from build123d import *

# Parameters (mm, degrees)
SKETCH1_W           = 42.418
SKETCH1_H           = 42.418
SKETCH1_R           = 3.175
BOSS_EXTRUDE1_DEPTH = 36.449
BOSS_EXTRUDE2_REACH = 68.815
SKETCH2_W           = 3.175
SKETCH2_H           = 42.418
SKETCH4_W           = 29.523081252
SKETCH4_H           = 25.4
CUT_EXTRUDE2_DEPTH  = 70.020848799
FILLET1_R           = 2.54
FILLET2_R           = 6.35


with BuildPart() as part:
    # Sketch1 → Boss-Extrude1 (new body)
    with BuildSketch(Plane.XY):
        with BuildLine():
            Line((4.064, -24.384), (24.384, -24.384))
            Line((24.384, -24.384), (24.384, 24.384))
            Line((24.384, 24.384), (4.064, 24.384))
            ThreePointArc((4.064, 24.384), (0, 32.512), (-4.064, 24.384))
            Line((-4.064, 24.384), (-24.384, 24.384))
            Line((-24.384, 24.384), (-24.384, -24.384))
            Line((-24.384, -24.384), (-4.064, -24.384))
            ThreePointArc((-4.064, -24.384), (0, -32.512), (4.064, -24.384))
        make_face()
        with BuildLine():
            ThreePointArc((-0.889, 24.384), (0, 30.607), (0.889, 24.384))
            Line((0.889, 24.384), (-0.889, 24.384))
        make_face(mode=Mode.SUBTRACT)
        Rectangle(SKETCH1_W, SKETCH1_H, mode=Mode.SUBTRACT)
        with Locations((0, -27.432)):
            Circle(SKETCH1_R, mode=Mode.SUBTRACT)
    extrude(amount=BOSS_EXTRUDE1_DEPTH)

    # Sketch2 → Boss-Extrude2 (add, up to next)
    with BuildSketch(Plane(origin=(-21.209, 0, 0), x_dir=(0, 0, -1), z_dir=(1, 0, 0)), mode=Mode.PRIVATE) as boss_extrude2_sk1:
        with Locations((-1.5875, 0)):
            Rectangle(SKETCH2_W, SKETCH2_H)
    boss_extrude2_tool1 = extrude(boss_extrude2_sk1.sketch, amount=BOSS_EXTRUDE2_REACH, mode=Mode.PRIVATE) - part.part
    add(boss_extrude2_tool1.solids().sort_by_distance((-21.209, 0, 1.5875))[0])

    # Sketch4 → Cut-Extrude2 (cut, through all)
    with BuildSketch(Plane(origin=(24.384, 0, 0), x_dir=(0, 0, -1), z_dir=(1, 0, 0))):
        with Locations((-21.687459374, 0)):
            Rectangle(SKETCH4_W, SKETCH4_H)
    extrude(amount=-CUT_EXTRUDE2_DEPTH, mode=Mode.SUBTRACT)

    # Fillet1
    fillet1_edges = [part.edges().sort_by_distance(p)[0] for p in [
        (-21.209, -21.209, 19.812),
        (21.209, -21.209, 19.812),
        (21.209, 21.209, 19.812),
        (-21.209, 21.209, 19.812),
        (24.384, 24.384, 18.2245),
        (24.384, -24.384, 18.2245),
        (-24.384, -24.384, 18.2245),
        (-24.384, 24.384, 18.2245),
        (22.7965, 12.7, 6.925918748),
        (22.7965, -12.7, 6.925918748),
        (-22.7965, 12.7, 6.925918748),
        (-22.7965, -12.7, 6.925918748),
    ]]
    fillet(fillet1_edges, radius=FILLET1_R)

    # Fillet2
    fillet2_edges = [part.edges().sort_by_distance(p)[0] for p in [
        (4.064, 24.384, 18.2245),
        (4.064, -24.384, 18.2245),
        (-4.064, -24.384, 18.2245),
        (-4.064, 24.384, 18.2245),
    ]]
    fillet(fillet2_edges, radius=FILLET2_R)


solid = part.part
For this review, take the finished solid that the model builds, in its own axes (mm). A direction names the side the tool comes from. Round coordinates to 2 decimals unless told otherwise and drop trailing zeros. Write each loop counter-clockwise with the first axis right and the second up, starting at its lowest first coordinate (ties: lowest second). Pieces come first, ordered by that corner, then holes. Notation, with made-up numbers: (72, 58) -> (119, 58) arc R28 ccw to (119, 89) -> close; hole circle Ø11 at (13.5, 45). An arc over 180 degrees is marked (long way). Use CSV: the item, a comma, the result in double quotes.
(1) Consider section D-D, the plane z = 4.5. Give the boundary of the cut face in (x, y) (3 decimals), plus the area to 3 significant figures.
Computed values:
outline,"(-24.384, -21.844) arc R2.54 ccw to (-21.844, -24.384) -> (-10.943, -24.384) arc R6.35 cw to (-4.863, -28.9) arc R5.08 ccw to (4.863, -28.9) arc R6.35 cw to (10.943, -24.384) -> (21.844, -24.384) arc R2.54 ccw to (24.384, -21.844) -> (24.384, 21.844) arc R2.54 ccw to (21.844, 24.384) -> (10.943, 24.384) arc R6.35 cw to (4.863, 28.9) arc R5.08 ccw to (-4.863, 28.9) arc R6.35 cw to (-10.943, 24.384) -> (-21.844, 24.384) arc R2.54 ccw to (-24.384, 21.844) -> close; hole (-21.209, -18.669) arc R2.54 ccw to (-18.669, -21.209) -> (18.669, -21.209) arc R2.54 ccw to (21.209, -18.669) -> (21.209, 18.669) arc R2.54 ccw to (18.669, 21.209) -> (-18.669, 21.209) arc R2.54 ccw to (-21.209, 18.669) -> close; hole circle Ø6.35 at (0, -27.432); hole (-0.889, 24.384) -> (0.889, 24.384) arc R3.175 ccw (long way) to start"
area,"684 mm²"
(2) Draft analysis for pull direction Y (two halves, no side actions). For faces 4 (the face through (-23.66, -23.62, 18.48)), 5 (the face through (-23, 0, 6.926)), 6 (the face through (0, -22, 36.449)), state which applies: +Y half, -Y half, draft (parallel to the pull), parting line (faces both ways), or undercut.
Computed values:
face 4,"-Y half"
face 5,"undercut"
face 6,"draft"
(3) Consider section C-C, the plane x = -16. Give the boundary of the cut face in (y, z) (3 decimals), plus the area to 3 significant figures.
Computed values:
outline,"(-24.384, 0) -> (24.384, 0) -> (24.384, 36.449) -> (21.209, 36.449) -> (21.209, 3.175) -> (-21.209, 3.175) -> (-21.209, 36.449) -> (-24.384, 36.449) -> close"
area,"366 mm²"
(4) Consider section A-A, the plane x = 0. Give the boundary of the cut face in (y, z) (3 decimals).
Computed values:
outline,"(-32.512, 0) -> (-30.607, 0) -> (-30.607, 36.449) -> (-32.512, 36.449) -> close; (-24.257, 0) -> (24.384, 0) -> (24.384, 36.449) -> (21.209, 36.449) -> (21.209, 3.175) -> (-21.209, 3.175) -> (-21.209, 36.449) -> (-24.257, 36.449) -> close; (30.607, 0) -> (32.512, 0) -> (32.512, 36.449) -> (30.607, 36.449) -> close"
(5) For faces 1 (the face through (0, 21.209, 20)), 2 (the face through (-16, 24.384, 18)), 3 (the face through (23, -12.7, 23)), list the 3-axis set-ups (+Z, -Z, +X, -X, +Y, -Y) from which the entire face can be reached by the end or side of a thin tool; tool diameter is ignored.
Computed values:
face 1,"+Z"
face 2,"+Z, -Z, -X, +Y"
face 3,"+Z, +X, -X"
(6) To check wall thickness, follow L1, parallel to X at y = -13, z = 24; L2, parallel to Z at x = 2, y = 15 (3 decimals). State the ranges of each line that lie inside material, in increasing order. Write a range as [from, to].
Computed values:
L1,"[-24.38, -21.21], [21.21, 24.38]"
L2,"[0, 3.175]"
(7) Consider section B-B, the plane y = 27.5. Give the boundary of the cut face in (x, z), plus the area to 3 significant figures.
Computed values:
outline,"(-5.48, 0) -> (-3.17, 0) -> (-3.17, 36.45) -> (-5.48, 36.45) -> close; (3.17, 0) -> (5.48, 0) -> (5.48, 36.45) -> (3.17, 36.45) -> close"
area,"168 mm²"
(8) Clearance check with flat-ended pins moving along their axes: P1, Ø3.5, axis at x = -19, z = 15, coming from the -Y side; P2, Ø5.5, axis at x = -17, z = 16, coming from the +Y side; P3, Ø1.6, axis at x = 23, y = 2, coming from the +Z side; P4, Ø7.5, axis at x = 0, y = -27.432, coming from the +Z side. State where each tip first meets the part, or that it passes through.
Computed values:
P1,"y = -24.38"
P2,"y = 24.38"
P3,"z = 6.93"
P4,"z = 36.45"
